from build123d import *

# Parameters (mm, degrees)
F0_R     = 1.5
F1_DEPTH = 2


with BuildPart() as f1:
    # F0 (on Top) → F1 (new body)
    with BuildSketch(Plane.XY):
        with BuildLine():
            ThreePointArc((-56.193922, 8.767486), (-55.315242, 6.646166), (-53.193922, 5.767486))
            Line((-53.193922, 5.767486), (-27.543922, 5.767486))
            ThreePointArc((-27.543922, 5.767486), (-25.422601, 6.646166), (-24.543922, 8.767486))
            Line((-24.543922, 8.767486), (-24.543922, 14.461119))
            ThreePointArc((-24.543922, 14.461119), (-24.785332, 15.995987), (-25.48625, 17.382643))
            Line((-25.48625, 17.382643), (-28.615086, 21.728248))
            ThreePointArc((-28.615086, 21.728248), (-32.104684, 22.296322), (-32.672758, 18.806724))
            Line((-32.672758, 18.806724), (-29.920853, 14.984635))
            ThreePointArc((-29.920853, 14.984635), (-29.640486, 14.429972), (-29.543922, 13.816025))
            Line((-29.543922, 13.816025), (-29.543922, 12.767486))
            ThreePointArc((-29.543922, 12.767486), (-30.129708, 11.353272), (-31.543922, 10.767486))
            Line((-31.543922, 10.767486), (-49.193922, 10.767486))
            ThreePointArc((-49.193922, 10.767486), (-50.608135, 11.353272), (-51.193922, 12.767486))
            Line((-51.193922, 12.767486), (-51.193922, 13.816024))
            ThreePointArc((-51.193922, 13.816024), (-51.097358, 14.429971), (-50.81699, 14.984633))
            Line((-50.81699, 14.984633), (-48.065085, 18.806724))
            ThreePointArc((-48.065085, 18.806724), (-48.633159, 22.296322), (-52.122757, 21.728248))
            Line((-52.122757, 21.728248), (-55.251593, 17.382643))
            ThreePointArc((-55.251593, 17.382643), (-55.952512, 15.995987), (-56.193922, 14.461119))
            Line((-56.193922, 14.461119), (-56.193922, 8.767486))
        make_face()
        with Locations((-53.693922, 15.267486)):
            Circle(F0_R, mode=Mode.SUBTRACT)
        with Locations((-50.093921, 20.267486)):
            Circle(F0_R, mode=Mode.SUBTRACT)
        with Locations((-27.043922, 15.267486)):
            Circle(F0_R, mode=Mode.SUBTRACT)
        with Locations((-30.643922, 20.267486)):
            Circle(F0_R, mode=Mode.SUBTRACT)
    extrude(amount=F1_DEPTH)


solid = f1.part
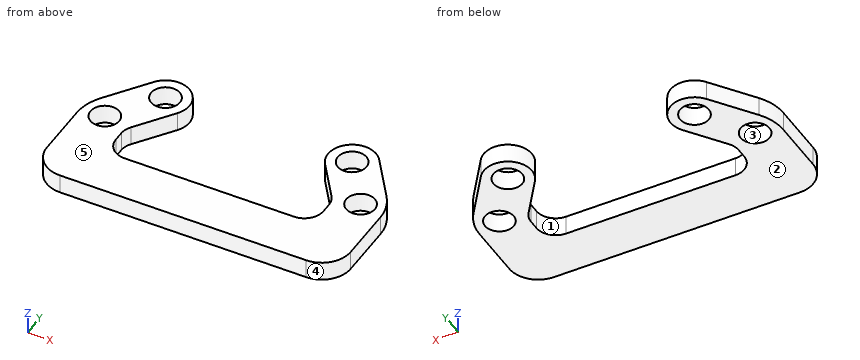
Check sheet for the modelled part. Datum: model origin and axes. Units: mm. Face numbers are marked on the shaded views. A direction names the side the tool comes from. Coordinates: 2 decimals unless noted, no trailing zeros. Loops run counter-clockwise (first coordinate to the right, second up) from the corner with the lowest first, then second, coordinate; pieces in that order, holes last. Notation, with made-up numbers: (-8.5, 79) -> (21.5, 79) arc R23 ccw to (21.5, 103) -> close; hole circle Ø5 at (79, -31.75). An arc over 180 degrees is marked (long way). Answer in a Markdown table with one row per item.
1. Sectioned sample at A-A, the plane y = 20.75. Record the boundary of the cut face in (x, z).
Check values:
| item | result |
|---|---|
| outline | (-52.83, 0) -> (-51.51, 0) -> (-51.51, 2) -> (-52.83, 2) -> close; (-48.67, 0) -> (-47.64, 0) -> (-47.64, 2) -> (-48.67, 2) -> close; (-33.1, 0) -> (-32.06, 0) -> (-32.06, 2) -> (-33.1, 2) -> close; (-29.22, 0) -> (-27.91, 0) -> (-27.91, 2) -> (-29.22, 2) -> close |
2. Sectioned sample at C-C, the plane z = 1.15. Record the boundary of the cut face in (x, y), then the cut area to 3 significant figures.
Check values:
| item | result |
|---|---|
| outline | (-56.19, 8.77) arc R3 ccw to (-53.19, 5.77) -> (-27.54, 5.77) arc R3 ccw to (-24.54, 8.77) -> (-24.54, 14.46) arc R5 ccw to (-25.49, 17.38) -> (-28.62, 21.73) arc R2.5 ccw to (-32.67, 18.81) -> (-29.92, 14.98) arc R2 cw to (-29.54, 13.82) -> (-29.54, 12.77) arc R2 cw to (-31.54, 10.77) -> (-49.19, 10.77) arc R2 cw to (-51.19, 12.77) -> (-51.19, 13.82) arc R2 cw to (-50.82, 14.98) -> (-48.07, 18.81) arc R2.5 ccw to (-52.12, 21.73) -> (-55.25, 17.38) arc R5 ccw to (-56.19, 14.46) -> close; hole circle Ø3 at (-53.69, 15.27); hole circle Ø3 at (-50.09, 20.27); hole circle Ø3 at (-30.64, 20.27); hole circle Ø3 at (-27.04, 15.27) |
| area | 254 mm2 |
3. Go/stop test with a flat-tipped pin: pin 1 (1 mm diameter, centred on x = -39, z = 1, fed in from +Y). Record where the tip stops, or that it passes through.
Check values:
| item | result |
|---|---|
| pin 1 | stops at y = 10.77 |
4. Material ranges on line 1 along X through (y, z) = (19, 1.2); line 2 along X through (y, z) = (15, 1.6); line 3 along Y through (x, z) = (-50.5, 1.7), recorded low to high. Write a range as [from, to].
Check values:
| item | result |
|---|---|
| line 1 | x = [-54.09, -50.9], [-49.29, -47.94], [-32.8, -31.45], [-29.84, -26.65] |
| line 2 | x = [-56.16, -55.17], [-52.22, -50.81], [-29.93, -28.52], [-25.57, -24.57] |
| line 3 | y = [5.77, 11.25], [15.42, 18.82], [21.71, 22.73] |
5. Sectioned sample at B-B, the plane x = -27. Record the boundary of the cut face in (y, z), then the cut area to 3 significant figures.
Check values:
| item | result |
|---|---|
| outline | (5.82, 0) -> (13.77, 0) -> (13.77, 2) -> (5.82, 2) -> close; (16.77, 0) -> (19.49, 0) -> (19.49, 2) -> (16.77, 2) -> close |
| area | 21.3 mm2 |
6. Release check for a two-part mould opening along Y. For the marked faces 3, 4 and 5 record: released by +Y, released by -Y, zero draft, split by the parting line, or undercut.
Check values:
| item | result |
|---|---|
| face 3 | undercut |
| face 4 | released by -Y |
| face 5 | zero draft |
7. Access from +Z, -Z, +X, -X, +Y, -Y to the whole of each face (thin tool, end or side, straight path). Record for the marked faces 1 and 2.
Check values:
| item | result |
|---|---|
| face 1 | +Z, -Z |
| face 2 | -Z, +X, -X, +Y, -Y |
8. Sectioned sample at D-D, the plane x = -46.5. Record the boundary of the cut face in (y, z).
Check values:
| item | result |
|---|---|
| outline | (5.77, 0) -> (10.77, 0) -> (10.77, 2) -> (5.77, 2) -> close |
